Print and shaded views of the part. All mm, measured from the part's lowest x, y and z. Coordinates: 2 decimals unless noted, no trailing zeros. Order: outer loops, then holes, each group sorted by start corner. A loop starts at its lowest first (then second) coordinate and runs counter-clockwise, first axis right, second up. Notation, with made-up numbers: M -4.75,-2 L 4.25,-2 A5 ccw 4.25,2 Z; hole C -31.5,82.5 d6. An arc over 180 degrees is marked long. One line per item, written item: value.
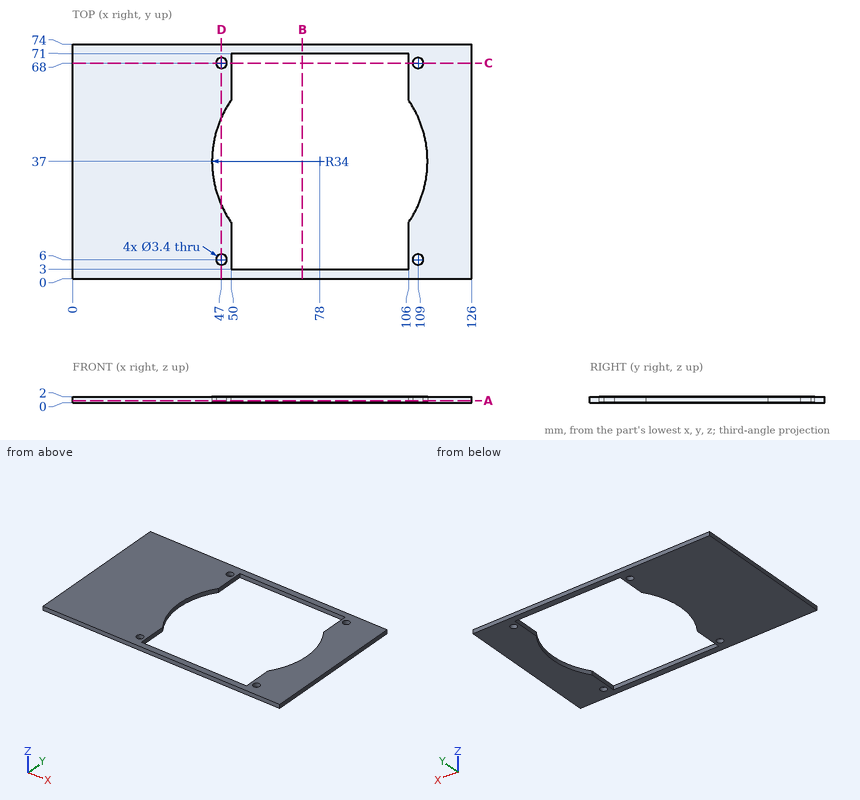
Q1. Slice it at B-B (x = 72.5). List the corners of the cut face in (y, z).
Recorded:
outline: M 0,0 L 3,0 L 3,2 L 0,2 Z; M 71,0 L 74,0 L 74,2 L 71,2 Z
Q2. Slice it at A-A (z = 0.7). List the corners of the cut face in (x, y), plus the area to 3 significant figures.
Recorded:
outline: M 0,0 L 126,0 L 126,74 L 0,74 Z; hole C 47,6 d3.4; hole C 47,68 d3.4; hole M 50,3 L 106,3 L 106,17.71 A34 ccw 106,56.29 L 106,71 L 50,71 L 50,56.29 A34 ccw 50,17.71 Z; hole C 109,6 d3.4; hole C 109,68 d3.4
area: 5,170 mm^2
Q3. Drill centre lines: line 1 along X through (y, z) = (68, 1.4); line 2 along X through (y, z) = (38, 0.5); line 3 along Y through (x, z) = (109, 0.85). Where is each one in solid material? Low to high.
Recorded:
line 1: x = 0 to 45.3, 48.7 to 50, 106 to 107.3, 110.7 to 126
line 2: x = 0 to 44.01, 111.99 to 126
line 3: y = 0 to 4.3, 7.7 to 23.04, 50.96 to 66.3, 69.7 to 74
Q4. Slice it at C-C (y = 68). List the corners of the cut face in (x, z), plus the area to 3 significant figures.
Recorded:
outline: M 0,0 L 45.3,0 L 45.3,2 L 0,2 Z; M 48.7,0 L 50,0 L 50,2 L 48.7,2 Z; M 106,0 L 107.3,0 L 107.3,2 L 106,2 Z; M 110.7,0 L 126,0 L 126,2 L 110.7,2 Z
area: 126 mm^2
Q5. Slice it at D-D (x = 47). List the corners of the cut face in (y, z).
Recorded:
outline: M 0,0 L 4.3,0 L 4.3,2 L 0,2 Z; M 7.7,0 L 23.04,0 L 23.04,2 L 7.7,2 Z; M 50.96,0 L 66.3,0 L 66.3,2 L 50.96,2 Z; M 69.7,0 L 74,0 L 74,2 L 69.7,2 Z
Q6. Pin check, flat tip, straight feed: pin 1 Ø3 at (x, y) = (109, 68) entering from +Z. Stop position of the tip, or through.
Recorded:
pin 1: passes through
